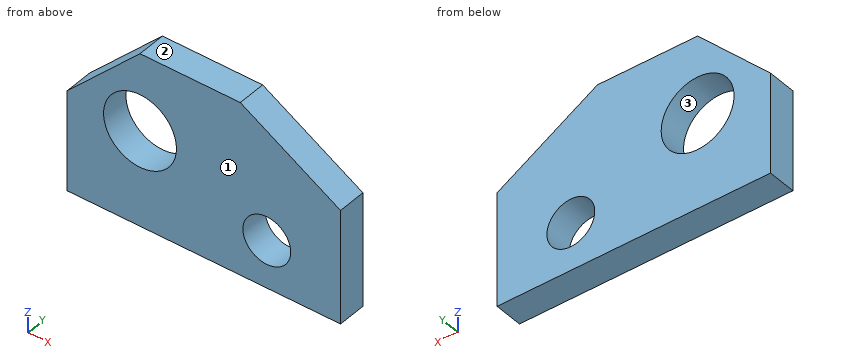
```python
from build123d import *

# Parameters (mm, degrees)
F0_R     = 21
F0_R_2   = 32
F1_DEPTH = 25


with BuildPart() as f1:
    # F0 (on Front) → F1 (new body)
    with BuildSketch(Plane.XZ):
        Polygon((-64, 4.07832), (-64, -83.92168), (176, -83.92168), (176, 16.07832), (88, 68.07832), (0, 68.07832), align=None)
        with Locations((111.296199, -42.076349)):
            Circle(F0_R, mode=Mode.SUBTRACT)
        Circle(F0_R_2, mode=Mode.SUBTRACT)
    extrude(amount=F1_DEPTH)


solid = f1.part
```
Work out the finished part from the listing and answer in its coordinate system (mm). Face numbers are marked on the shaded views. Coordinates: 2 decimals unless noted, no trailing zeros. Write each loop counter-clockwise with the first axis right and the second up, starting at its lowest first coordinate (ties: lowest second). Pieces come first, ordered by that corner, then holes. Notation, with made-up numbers: (85.25, 36.5) - (142.25, 36.5) arc R12 cw to (142.25, 46.5) - close; hole circle Ø7 at (25, 82). An arc over 180 degrees is marked (long way). Answer as a JSON object with one key per item and string values.
Q1. For a pull along Z with two mould halves and no side action, classify the marked faces 1, 2 and 3 as pulls with the +Z half, pulls with the -Z half, needs draft (parallel to the pull), parting line crosses it, or undercut.
Results list:
{"face 1": "needs draft", "face 2": "pulls with the +Z half", "face 3": "undercut"}
Q2. Consider L1, parallel to Z at x = 0, y = -17.5; L2, parallel to Z at x = 19, y = -18.5; L3, parallel to X at y = -9, z = -12. Determine where each line is inside the solid, lowest interval first. Write a range as from..to.
Results list:
{"L1": "z = -83.92..-32, 32..68.08", "L2": "z = -83.92..-25.75, 25.75..68.08", "L3": "x = -64..-29.66, 29.66..176"}
Q3. Find section A-A (z = 0). Write down the section's boundary in (x, y).
Results list:
{"outline": "(-64, -25) - (-32, -25) - (-32, 0) - (-64, 0) - close; (32, -25) - (176, -25) - (176, 0) - (32, 0) - close"}
Q4. Find section B-B (x = 19.5). Write down the section's boundary in (y, z).
Results list:
{"outline": "(-25, -83.92) - (0, -83.92) - (0, -25.37) - (-25, -25.37) - close; (-25, 25.37) - (0, 25.37) - (0, 68.08) - (-25, 68.08) - close"}
Q5. Given pin 1 Ø8 at (y, z) = (-13, 17) entering from +X; pin 2 Ø2 at (y, z) = (-19, 29.5) entering from +X; pin 3 Ø3 at (y, z) = (-13, 36.5) entering from +X, each flat-ended and moving along its own axis, determine where each tip first touches the part or whether it passes through.
Results list:
{"pin 1": "stops at x = 176", "pin 2": "stops at x = 154.98", "pin 3": "stops at x = 143.98"}
Q6. Find section C-C (y = -9.5). Write down the section's boundary in (x, z), plus the area to 3 significant figures.
Results list:
{"outline": "(-64, -83.92) - (176, -83.92) - (176, 16.08) - (88, 68.08) - (0, 68.08) - (-64, 4.08) - close; hole circle Ø64 at (0, 0); hole circle Ø42 at (111.3, -42.08)", "area": "27,500 mm^2"}
